Model file for the job. Use its own axes, mm. Face numbers are marked on the shaded views. A direction names the side the tool comes from. Give positions to 0.01 mm unless a question says otherwise; leave off trailing zeros. Write each loop counter-clockwise with the first axis right and the second up, starting at its lowest first coordinate (ties: lowest second). Pieces come first, ordered by that corner, then holes. Notation, with made-up numbers: M 64.25,14 L 94.25,14 A36 ccw 94.25,48 Z; hole C -14,-26 d3. An arc over 180 degrees is marked long. Answer as a JSON object with one key per item and string values. Group by question number.
Autodesk Inventor part; units mm, degrees
ref_plane "YZ Plane" through (0, 0, 0) normal (1, 0, 0) x (0, 1, 0)
ref_plane "XZ Plane" through (0, 0, 0) normal (0, 1, 0) x (-1, 0, 0)
ref_plane "XY Plane" through (0, 0, 0) normal (0, 0, 1) x (1, 0, 0)
sketch "Sketch1" plane through (0, 0, 0) normal (0, 1, 0) x (-1, 0, 0)
  point P0 (0, 0)
sketch "Sketch2" plane through (0, 0, 0) normal (0, 1, 0) x (-1, 0, 0)
  circle A0 centre (0, 0) radius 6
  dimension "d20" = 12
extrude "Extrusion1" add sketch "Sketch2" along normal blind 50
ref_plane "Work Plane1" through (0, 48, 0) normal (0, 1, 0) x (1, 0, 0)
sketch "Sketch3" plane through (0, 48, 0) normal (0, 1, 0) x (1, 0, 0)
  line L0 (0, 0) -> (2, 0)
  circle A0 centre (2, 0) radius 10
  dimension "d4" = 2
  dimension "d5" = 20
extrude "Extrusion2" add sketch "Sketch3" against normal blind 3
ref_plane "Work Plane2" through (2, 43, 0) normal (0, -1, 0) x (1, 0, 0)
sketch "Sketch5" plane through (2, 43, 0) normal (0, -1, 0) x (1, 0, 0)
  line L0 (-2, 0) -> (-4, 0)
  circle A0 centre (-4, 0) radius 10
  dimension "d16" = 2
  dimension "d17" = 20
extrude "Extrusion4" add sketch "Sketch5" along normal blind 3
sketch "Sketch6" plane through (0, 0, 0) normal (0, -1, 0) x (1, 0, 0)
  circle A0 centre (0, 0) radius 3.5
  arc A1 (4.2426, 1.5) -> (4.2426, -1.5) centre (0, 0) ccw
  line L0 (5.4, 1.5) -> (4.2426, 1.5)
  line L1 (4.2426, -1.5) -> (5.4, -1.5)
  line L2 (5.4, -1.5) -> (5.4, 1.5)
  point P0 (0, 0)
  point P1 (0, 0)
extrude "Extrusion5" cut sketch "Sketch6" against normal blind 4 contours A0 | L0 L2 L1 A1
fillet "Fillet1" radius 1 1 edges at (-4.5, 0, 0)
properties part number "input_shaft"
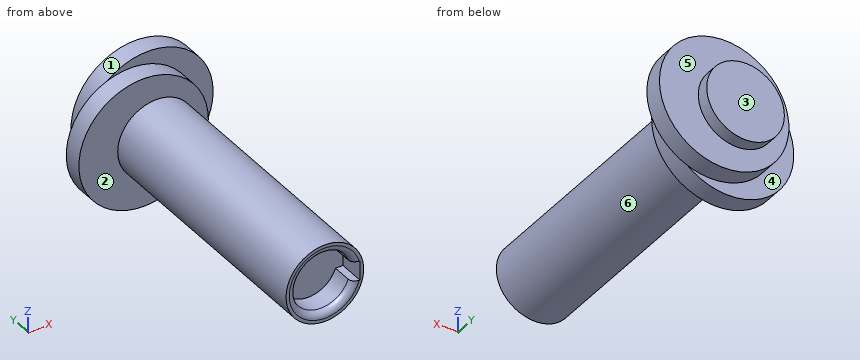
Q1. Slice it at C-C, the plane z = -8.25. Write the cut outline in (x, y), then the cut area to 3 significant figures.
Q2. Slice it at B-B, the plane x = -6.5. Write the cut outline in (y, z), then the cut area to 3 significant figures.
Q3. 3-axis set-ups, long thin cutter, end or side, ignore diameter. For the marked faces 1, 2 and 3: which of +Z, -Z, +X, -X, +Y, -Y reach the whole face in a straight line?
Q4. Two-plate mould, pull along Y, no slides. Class the marked faces 4, 5 and 6: +Y half, -Y half, draft (parallel to the pull), parting line (faces both ways), or undercut.
Q5. Wall check: L1, parallel to Z at x = 0, y = 3.1; L2, parallel to X at y = 1.8, z = 0; L3, parallel to Y at x = -1.5, z = -8.25. Give the ranges that are in metal, low to high.
Q6. Drop flat-ended pins along their axis: P1, Ø6, axis at y = 19, z = -6.5, coming from the +X side; P2, Ø10, axis at x = -2, z = 0, coming from the -Y side; P3, Ø1, axis at x = 5, z = 4.5, coming from the -Y side; P4, Ø4, axis at x = 0, z = -0.5, coming from the -Y side. Give the stop position or say it passes through.
Q7. Slice it at A-A, the plane z = 0. Write the cut outline in (x, y).
Q8. Slice it at D-D, the plane x = 0. Write the cut outline in (y, z).
Solved:
{
 "1": {"outline": "M -7.65,40 L 3.65,40 L 3.65,43 L -7.65,43 Z; M -3.65,45 L 7.65,45 L 7.65,48 L -3.65,48 Z", "area": "67.8 mm²"},
 "2": {"outline": "M 40,-8.93 L 43,-8.93 L 43,8.93 L 40,8.93 Z; M 45,-5.27 L 48,-5.27 L 48,5.27 L 45,5.27 Z", "area": "85.2 mm²"},
 "3": {"face 1": "+Y", "face 2": "-Y", "face 3": "+Z, -Z, +X, -X, +Y"},
 "4": {"face 4": "undercut", "face 5": "+Y half", "face 6": "draft"},
 "5": {"L1": "z = -6 to -4.5, 4.5 to 6", "L2": "x = -6 to -4.5, 5.4 to 6", "L3": "y = 40 to 43, 45 to 48"},
 "6": {"P1": "stops at x = 4.87", "P2": "stops at y = 0", "P3": "stops at y = 40", "P4": "stops at y = 4"},
 "7": {"outline": "M -12,40 L -6,40 L -6,0 L -5.5,0 A1 ccw -4.5,1 L -4.5,4 L 5.4,4 L 5.4,0 L 6,0 L 6,40 L 8,40 L 8,43 L 6,43 L 6,45 L 12,45 L 12,48 L 6,48 L 6,50 L -6,50 L -6,48 L -8,48 L -8,45 L -6,45 L -6,43 L -12,43 Z"},
 "8": {"outline": "M 0,-6 L 40,-6 L 40,-9.8 L 43,-9.8 L 43,-6 L 45,-6 L 45,-9.8 L 48,-9.8 L 48,-6 L 50,-6 L 50,6 L 48,6 L 48,9.8 L 45,9.8 L 45,6 L 43,6 L 43,9.8 L 40,9.8 L 40,6 L 0,6 L 0,5.5 A1 ccw 1,4.5 L 4,4.5 L 4,-4.5 L 1,-4.5 A1 ccw 0,-5.5 Z"}
}
